from build123d import *

# Parameters (mm, degrees)
F0_W     = 6
F0_H     = 5
F0_W_2   = 1.2
F1_DEPTH = 1.2
F2_DEPTH = 5
F3_DEPTH = 10
F5_DEPTH = 65
F6_DEPTH = 10


with BuildPart() as f1:
    # F0 (on Top) → F1 (new body)
    with BuildSketch(Plane.XY):
        with Locations((14.2, -2.5)):
            Rectangle(F0_W, F0_H)
        with Locations((10.6, -2.5)):
            Rectangle(F0_W_2, F0_H)
        Polygon((10, 0), (0, 0), (0, -76.2), (78.9, -76.2), (78.9, 0), (68.9, 0), (68.9, -5), (67.7, -5), (61.7, -5), (61.7, 0), (17.2, 0), (17.2, -5), (11.2, -5), (10, -5), align=None)
        Polygon((10, -60), (11.2, -60), (17.2, -60), (17.2, -65), (17.2, -66.2), (10, -66.2), align=None, mode=Mode.SUBTRACT)
        Polygon((61.7, -65), (61.7, -60), (67.7, -60), (68.9, -60), (68.9, -66.2), (61.7, -66.2), align=None, mode=Mode.SUBTRACT)
        with Locations((64.7, -2.5)):
            Rectangle(F0_W, F0_H)
        with Locations((68.3, -2.5)):
            Rectangle(F0_W_2, F0_H)
        with Locations((64.7, -62.5)):
            Rectangle(F0_W, F0_H)
        Polygon((68.9, -60), (67.7, -60), (67.7, -65), (61.7, -65), (61.7, -66.2), (68.9, -66.2), align=None)
        with Locations((14.2, -62.5)):
            Rectangle(F0_W, F0_H)
        Polygon((11.2, -65), (11.2, -60), (10, -60), (10, -66.2), (17.2, -66.2), (17.2, -65), align=None)
    extrude(amount=-F1_DEPTH)

    # F0 (on Top) → F2 (join)
    with BuildSketch(Plane.XY):
        with Locations((14.2, -2.5)):
            Rectangle(F0_W, F0_H)
        with Locations((14.2, -62.5)):
            Rectangle(F0_W, F0_H)
        with Locations((64.7, -2.5)):
            Rectangle(F0_W, F0_H)
        with Locations((64.7, -62.5)):
            Rectangle(F0_W, F0_H)
    extrude(amount=F2_DEPTH)

    # F0 (on Top) → F3 (join)
    with BuildSketch(Plane.XY):
        Polygon((11.2, -65), (11.2, -60), (10, -60), (10, -66.2), (17.2, -66.2), (17.2, -65), align=None)
        Polygon((68.9, -60), (67.7, -60), (67.7, -65), (61.7, -65), (61.7, -66.2), (68.9, -66.2), align=None)
        with Locations((68.3, -2.5)):
            Rectangle(F0_W_2, F0_H)
        with Locations((10.6, -2.5)):
            Rectangle(F0_W_2, F0_H)
    extrude(amount=F3_DEPTH)

    # F4 (on face) → F5 (join, through all)
    with BuildSketch(Plane(origin=(0, 0, 0), x_dir=(-1, 0, 0), z_dir=(0, 1, 0))):
        Polygon((-11.2, 6), (-11.2, 10), (-12.7, 8.5), (-12.7, 7.5), align=None)
        Polygon((-66.2, 7.5), (-66.2, 8.5), (-67.7, 10), (-67.7, 6), align=None)
    extrude(amount=-F5_DEPTH)

    # F0 (on Top) → F6 (cut, through all)
    with BuildSketch(Plane.XY):
        Polygon((10, 0), (0, 0), (0, -76.2), (78.9, -76.2), (78.9, 0), (68.9, 0), (68.9, -5), (67.7, -5), (61.7, -5), (61.7, 0), (17.2, 0), (17.2, -5), (11.2, -5), (10, -5), align=None)
        Polygon((10, -60), (11.2, -60), (17.2, -60), (17.2, -65), (17.2, -66.2), (10, -66.2), align=None, mode=Mode.SUBTRACT)
        Polygon((61.7, -65), (61.7, -60), (67.7, -60), (68.9, -60), (68.9, -66.2), (61.7, -66.2), align=None, mode=Mode.SUBTRACT)
    extrude(amount=F6_DEPTH, mode=Mode.SUBTRACT)


solid = f1.part
The listing builds one solid part. Answer for the finished solid, in the listing's coordinates (mm). A direction names the side the tool comes from. Round coordinates to 2 decimals unless told otherwise and drop trailing zeros. Write each loop counter-clockwise with the first axis right and the second up, starting at its lowest first coordinate (ties: lowest second). Pieces come first, ordered by that corner, then holes. Notation, with made-up numbers: (41.5, 26) - (73.5, 26) arc R20 cw to (73.5, 47) - close; hole circle Ø1 at (70, 27.5). An arc over 180 degrees is marked (long way). Use a Markdown table: item, result. Add a question column.
1. The part is cut by section A-A (x = 33). Write down the section's boundary in (y, z), and give its area (3 significant figures).
2. For a pull along X with two mould halves and no side action, classify faces 6 (the face through (14, -62, 5)), 7 (the face through (68.9, -63, 5)), 8 (the face through (10, -3, 5)) as +X half, -X half, draft (parallel to the pull), parting line (faces both ways), or undercut.
3. The part is cut by section B-B (y = -53). Write down the section's boundary in (x, z).
4. A tool of negligible diameter and unlimited length cuts with its end or side. For faces 1 (the face through (10, -63, 5)), 2 (the face through (17.2, -3, 2)), 3 (the face through (65, -66.2, 5)), 4 (the face through (66, -5, 4)), 5 (the face through (65, -2, 5)), from which of +Z, -Z, +X, -X, +Y, -Y can it reach the whole face along a straight path? Write none if from no direction.
5. Consider line 1 (Y direction, x = 14, z = 0.75); line 2 (Z direction, x = 47.5, y = -25.5); line 3 (Y direction, x = 63, z = 8.75). Determine where each line is inside the solid, lowest interval first.
6. Flat-ended cylindrical pins translate along their axes: P1, Ø3, axis at y = -61.5, z = 6, coming from the -X side; P2, Ø1.5, axis at x = 14, y = -62, coming from the +Z side; P3, Ø6, axis at x = 24, z = 4, coming from the +Y side; P4, Ø1.5, axis at y = -3.5, z = 2.5, coming from the +X side. Find the tip coordinate at first contact, or state that the pin passes through.
Reported:
| question | item | result |
|---|---|---|
| 1 | outline | (-76.2, -1.2) - (0, -1.2) - (0, 0) - (-76.2, 0) - close |
| 1 | area | 91.4 mm^2 |
| 2 | face 6 | undercut |
| 2 | face 7 | +X half |
| 2 | face 8 | -X half |
| 3 | outline | (0, -1.2) - (78.9, -1.2) - (78.9, 0) - (0, 0) - close |
| 4 | face 1 | +Z, -X, +Y, -Y |
| 4 | face 2 | +Z, +Y, -Y |
| 4 | face 3 | +Z, +X, -X, -Y |
| 4 | face 4 | +Z, +X, -X |
| 4 | face 5 | +Y |
| 5 | line 1 | -66.2 to -60, -5 to 0 |
| 5 | line 2 | -1.2 to 0 |
| 5 | line 3 | -66.2 to -65 |
| 6 | P1 | x = 10 |
| 6 | P2 | z = 5 |
| 6 | P3 | through |
| 6 | P4 | x = 68.9 |
